Could you check a few things on this model? Use its own coordinates, in mm. Coordinates: 2 decimals unless noted, no trailing zeros. Order: outer loops, then holes, each group sorted by start corner. A loop starts at its lowest first (then second) coordinate and runs counter-clockwise, first axis right, second up. Notation, with made-up numbers: (33, 11.25) - (42, 11.25) arc R18 cw to (42, 30.25) - close; hole circle Ø6 at (12, 47). An arc over 180 degrees is marked (long way). Answer as a JSON object with one key per item and string values. Group by question number.
(1) Please list where these lines run through material, in increasing order: probe 1 along Y at (x, z) = (35, -1.7); probe 2 along X at (y, z) = (9, -1.5); probe 3 along X at (y, z) = (12, -3.1).
(2) Imagine slicing it at B-B, the plane x = -35. Write out the boundary of the cut face in (y, z).
(3) Imagine slicing it at C-C, the plane z = -4.1. Write out the boundary of the cut face in (x, y), and give its area (3 significant figures).
(4) Imagine slicing it at D-D, the plane y = -15. Write out the boundary of the cut face in (x, z).
(5) Imagine slicing it at A-A, the plane y = -3.5. Write out the boundary of the cut face in (x, z), and give its area (4 significant figures).
(6) Will these pins go through, and if not, where does the flat tip stop? P1, Ø6, axis at x = -35, y = -15, coming from the +Z side (3 decimals); P2, Ø11.5, axis at x = 35, y = 15, coming from the +Z side.
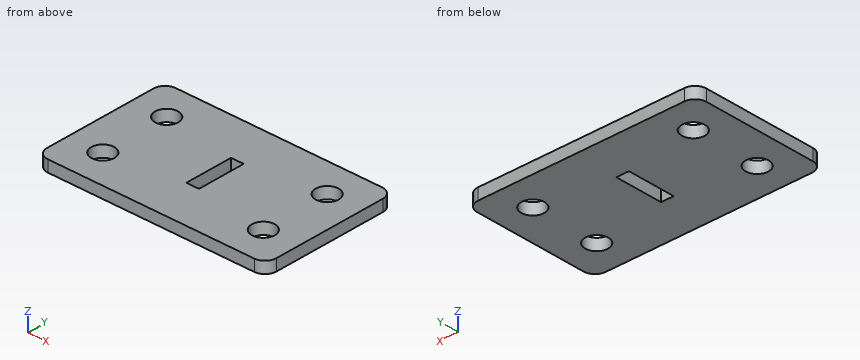
from build123d import *

# Parameters (mm, degrees)
IZIM1_W               = 100
IZIM1_H               = 60
TABAN_FLAN_1_DEPTH    = 5
RADYUS1_R             = 5
IZIM6_R               = 5
KES_EKSTR_ZYON1_DEPTH = 10
IZIM7_W               = 5.5
IZIM7_H               = 21
KES_EKSTR_ZYON2_DEPTH = 10


# Sheet-metal steps are written as plain solids
with BuildPart() as part:
    # Çizim1 → Taban-Flanş1 (new body)
    with BuildSketch(Plane.XY):
        Rectangle(IZIM1_W, IZIM1_H)
    extrude(amount=-TABAN_FLAN_1_DEPTH)

    # Radyus1
    radyus1_edges = [part.edges().sort_by_distance(p)[0] for p in [
        (50, -30, -2.5),
        (-50, -30, -2.5),
        (-50, 30, -2.5),
        (50, 30, -2.5),
    ]]
    fillet(radyus1_edges, radius=RADYUS1_R)

    # Çizim6 → Kes-Ekstrüzyon1 (cut)
    with BuildSketch(Plane.XY):
        with Locations((-35, 15)):
            Circle(IZIM6_R)
        with Locations((-35, -15)):
            Circle(IZIM6_R)
        with Locations((35, 15)):
            Circle(IZIM6_R)
        with Locations((35, -15)):
            Circle(IZIM6_R)
    extrude(amount=-KES_EKSTR_ZYON1_DEPTH, mode=Mode.SUBTRACT)

    # Çizim7 → Kes-Ekstrüzyon2 (cut)
    with BuildSketch(Plane(origin=(0, 0, -5), x_dir=(-1, 0, 0), z_dir=(0, 0, -1))):
        Rectangle(IZIM7_W, IZIM7_H)
    extrude(amount=-KES_EKSTR_ZYON2_DEPTH, mode=Mode.SUBTRACT)


solid = part.part
Result set:
{
 "1": {"probe 1": "y = -30 to -20, -10 to 10, 20 to 30", "probe 2": "x = -50 to -2.75, 2.75 to 50", "probe 3": "x = -50 to -39, -31 to 31, 39 to 50"},
 "2": {"outline": "(-30, -5) - (-20, -5) - (-20, 0) - (-30, 0) - close; (-10, -5) - (10, -5) - (10, 0) - (-10, 0) - close; (20, -5) - (30, -5) - (30, 0) - (20, 0) - close"},
 "3": {"outline": "(-50, -25) arc R5 ccw to (-45, -30) - (45, -30) arc R5 ccw to (50, -25) - (50, 25) arc R5 ccw to (45, 30) - (-45, 30) arc R5 ccw to (-50, 25) - close; hole circle Ø10 at (-35, -15); hole circle Ø10 at (-35, 15); hole (-2.75, -10.5) - (2.75, -10.5) - (2.75, 10.5) - (-2.75, 10.5) - close; hole circle Ø10 at (35, -15); hole circle Ø10 at (35, 15)", "area": "5,550 mm^2"},
 "4": {"outline": "(-50, -5) - (-40, -5) - (-40, 0) - (-50, 0) - close; (-30, -5) - (30, -5) - (30, 0) - (-30, 0) - close; (40, -5) - (50, -5) - (50, 0) - (40, 0) - close"},
 "5": {"outline": "(-50, -5) - (-2.75, -5) - (-2.75, 0) - (-50, 0) - close; (2.75, -5) - (50, -5) - (50, 0) - (2.75, 0) - close", "area": "472.5 mm^2"},
 "6": {"P1": "passes through", "P2": "stops at z = 0"}
}
